Model file for the job. Use its own axes, mm. A direction names the side the tool comes from. Round coordinates to 2 decimals unless told otherwise and drop trailing zeros. Write each loop counter-clockwise with the first axis right and the second up, starting at its lowest first coordinate (ties: lowest second). Pieces come first, ordered by that corner, then holes. Notation, with made-up numbers: (1.5, 16) - (11.5, 16) arc R15 ccw to (11.5, 23) - close; hole circle Ø11 at (-34, 33.5). An arc over 180 degrees is marked (long way). One line per item, written item: value.
from build123d import *

# Parameters (mm, degrees)
M16_TAPPED_HOLE1_D     = 14
M16_TAPPED_HOLE1_DEPTH = 42
CHAMFER1_SIZE          = 2


with BuildPart() as part:
    # Sketch1 → Revolve1 (revolve)
    with BuildSketch(Plane.XY, mode=Mode.PRIVATE) as revolve1_sk:
        Polygon((0, 36), (0, 11), (45, 11), (45, 0), (60, 0), (60, 19), (57, 22), (35, 22), (35, 33), (32, 36), align=None)
    revolve(revolve1_sk.sketch.rotate(Axis((0, 0, 0), (0, 1, 0)), 90), axis=Axis((0, 0, 0), (0, 1, 0)))

    # M16 Tapped Hole1
    with Locations(Plane(origin=(0, 36, 0), x_dir=(1, 0, 0), z_dir=(0, 1, 0))):
        with Locations((0, 0)):
            Hole(M16_TAPPED_HOLE1_D / 2, depth=M16_TAPPED_HOLE1_DEPTH)

    # Chamfer1
    chamfer1_edges = [part.edges().sort_by_distance(p)[0] for p in [
        (7, 36, 0),
    ]]
    chamfer(chamfer1_edges, length=CHAMFER1_SIZE)


solid = part.part
1. Band-saw the part on C-C on y = 3.5. Write the cut outline in (x, z).
Report:
outline: circle Ø120 at (0, 0); hole circle Ø90 at (0, 0)
2. Wall check: probe 1 along X at (y, z) = (25.75, 0); probe 2 along X at (y, z) = (8.75, 0). Give the ranges that are in metal, low to high. Write a range as [from, to].
Report:
probe 1: [-35, -7], [7, 35]
probe 2: [-60, -45], [45, 60]
3. Mould opens along X. For faces 1 (the face through (-6.466, 22.339, 2.681)), 2 (the face through (-50.59, 9.63, -32.26)), 3 (the face through (7, 36, -7)) say: released by +X, released by -X, zero draft, split by the parting line, or undercut.
Report:
face 1: undercut
face 2: split by the parting line
face 3: zero draft
4. Band-saw the part on A-A on x = 0. Write the cut outline in (y, z).
Report:
outline: (0, -60) - (19, -60) - (22, -57) - (22, -35) - (33, -35) - (36, -32) - (36, -9) - (34, -7) - (11, -7) - (11, -45) - (0, -45) - close; (0, 45) - (11, 45) - (11, 7) - (34, 7) - (36, 9) - (36, 32) - (33, 35) - (22, 35) - (22, 57) - (19, 60) - (0, 60) - close
5. Band-saw the part on B-B on z = 0. Write the cut outline in (x, y), plus the area to 3 significant figures.
Report:
outline: (-60, 0) - (-45, 0) - (-45, 11) - (-7, 11) - (-7, 34) - (-9, 36) - (-32, 36) - (-35, 33) - (-35, 22) - (-57, 22) - (-60, 19) - close; (7, 11) - (45, 11) - (45, 0) - (60, 0) - (60, 19) - (57, 22) - (35, 22) - (35, 33) - (32, 36) - (9, 36) - (7, 34) - close
area: 2,260 mm²
6. Drop flat-ended pins along their axis: pin 1 (16 mm diameter, centred on x = 0, z = 0, fed in from -Y); pin 2 (3 mm diameter, centred on x = 4, z = -36, fed in from +Y); pin 3 (4 mm diameter, centred on y = 8.5, z = 9, fed in from -X). Give the stop position or say it passes through.
Report:
pin 1: y = 11
pin 2: y = 33.28
pin 3: x = -59.59
7. Tool access for faces 4 (the face through (-45, 0, 9)), 5 (the face through (-26, 22, -25)), 6 (the face through (39.923, 5.423, -20.765)): list every direction of +Z, -Z, +X, -X, +Y, -Y with a clear straight run to the whole face (end or side of a thin tool).
Report:
face 4: +Z, -Z, +X, -X, -Y
face 5: +Y
face 6: -Y
8. Band-saw the part on D-D on y = 27.5. Write the cut outline in (x, z).
Report:
outline: circle Ø70 at (0, 0); hole circle Ø14 at (0, 0)
